from build123d import *

# Parameters (mm, degrees)
SKETCH_1_W          = 80
SKETCH_1_H          = 90
SKETCH_1_R          = 3
SKETCH_1_R_2        = 2
SKETCH_1_W_2        = 20
SKETCH_1_H_2        = 41
EXTRUDE_1_DEPTH     = 5
FILLET_1_R          = 10
SKETCH_2_R          = 1.5
CUT_EXTRUDE_1_DEPTH = 73.284161474


with BuildPart() as part:
    # 草图1 → 凸台-拉伸1 (new body)
    with BuildSketch(Plane(origin=(0, 0, 0), x_dir=(1, 0, 0), z_dir=(0, 1, 0))):
        with Locations((0, 15)):
            Rectangle(SKETCH_1_W, SKETCH_1_H)
        with Locations(Location((27.5, 15, 0), (0, 0, 270))):
            Circle(SKETCH_1_R, mode=Mode.SUBTRACT)
        with Locations(Location((27.5, -15, 0), (0, 0, 270))):
            Circle(SKETCH_1_R, mode=Mode.SUBTRACT)
        with Locations(Location((-27.5, -15, 0), (0, 0, 90))):
            Circle(SKETCH_1_R, mode=Mode.SUBTRACT)
        with Locations(Location((-27.5, 15, 0), (0, 0, 90))):
            Circle(SKETCH_1_R, mode=Mode.SUBTRACT)
        with Locations(Location((4.95, 24.3, 0), (0, 0, 270))):
            Circle(SKETCH_1_R_2, mode=Mode.SUBTRACT)
        with Locations(Location((-4.95, 24.3, 0), (0, 0, 90))):
            Circle(SKETCH_1_R_2, mode=Mode.SUBTRACT)
        with Locations(Location((4.95, -24.3, 0), (0, 0, 90))):
            Circle(SKETCH_1_R_2, mode=Mode.SUBTRACT)
        with Locations(Location((-4.95, -24.3, 0), (0, 0, 270))):
            Circle(SKETCH_1_R_2, mode=Mode.SUBTRACT)
        with Locations(Location((-27.5, 45, 0), (0, 0, 90))):
            Circle(SKETCH_1_R, mode=Mode.SUBTRACT)
        with Locations(Location((27.5, 45, 0), (0, 0, 270))):
            Circle(SKETCH_1_R, mode=Mode.SUBTRACT)
        Rectangle(SKETCH_1_W_2, SKETCH_1_H_2, mode=Mode.SUBTRACT)
    extrude(amount=EXTRUDE_1_DEPTH)

    # 圆角1
    fillet_1_edges = [part.edges().sort_by_distance(p)[0] for p in [
        (40, 2.5, -60),
        (40, 2.5, 30),
        (-40, 2.5, 30),
        (-40, 2.5, -60),
    ]]
    fillet(fillet_1_edges, radius=FILLET_1_R)

    # 草图2 → 切除-拉伸1 (cut, through all)
    with BuildSketch(Plane(origin=(0, 0, 0), x_dir=(1, 0, 0), z_dir=(0, 1, 0))):
        with Locations(Location((0, 54.15, 0), (0, 0, 270))):
            Circle(SKETCH_2_R)
        with Locations(Location((8, 46.15, 0), (0, 0, 270))):
            Circle(SKETCH_2_R)
        with Locations(Location((0, 38.15, 0), (0, 0, 270))):
            Circle(SKETCH_2_R)
        with Locations(Location((-8, 46.15, 0), (0, 0, 270))):
            Circle(SKETCH_2_R)
    extrude(amount=CUT_EXTRUDE_1_DEPTH, mode=Mode.SUBTRACT)


solid = part.part
The model under review builds one solid part; all positions refer to its coordinate system, in mm. A direction names the side the tool comes from. Round coordinates to 2 decimals unless told otherwise and drop trailing zeros. Write each loop counter-clockwise with the first axis right and the second up, starting at its lowest first coordinate (ties: lowest second). Pieces come first, ordered by that corner, then holes. Notation, with made-up numbers: M -37.75,53 L 20.25,53 A23 ccw 20.25,78 Z; hole C 10,-7 d4. An arc over 180 degrees is marked long. Answer as CSV lines item,"result". Start each with the question number.
Q1. Consider section B-B, the plane z = -24.3. Give the boundary of the cut face in (x, y), then the cut area to 3 significant figures.
Q2. Consider section D-D, the plane x = -8. Give the boundary of the cut face in (y, z), then the cut area to 3 significant figures.
Q3. Consider section A-A, the plane x = 27.5. Give the boundary of the cut face in (y, z).
Q4. Consider section C-C, the plane y = 3.05. State how many separate pieces and enclosed holes the cut face has, then the cut area to 3 significant figures.
Q5. The part is to be moulded in two halves that separate along X. For faces 1 (the face through (0, 2, 30)), 2 (the face through (-27.6, 2.5, -12)), 3 (the face through (-40, 2, -15)), say which applies: +X half, -X half, draft (parallel to the pull), parting line (faces both ways), or undercut.
Q6. Wall thickness on line 1 along Z through (x, y) = (-8, 2.1); line 2 along X through (y, z) = (2.2, -15); line 3 along Z through (x, y) = (0, 3.7): over which ranges is each line inside the solid? List them lowest first.
Q7. Tool access review of faces 4 (the face through (0, 2, -20.5)), 5 (the face through (40, 2, -15)): name each direction out of +Z, -Z, +X, -X, +Y, -Y from which nothing blocks a thin tool from reaching the whole face with its end or side.
Result set:
1,outline,"M -40,0 L -6.95,0 L -6.95,5 L -40,5 Z; M -2.95,0 L 2.95,0 L 2.95,5 L -2.95,5 Z; M 6.95,0 L 40,0 L 40,5 L 6.95,5 Z"
1,area,"360 mm²"
2,outline,"M 0,-60 L 5,-60 L 5,-47.65 L 0,-47.65 Z; M 0,-44.65 L 5,-44.65 L 5,-20.5 L 0,-20.5 Z; M 0,20.5 L 5,20.5 L 5,30 L 0,30 Z"
2,area,"230 mm²"
3,outline,"M 0,-60 L 5,-60 L 5,-48 L 0,-48 Z; M 0,-42 L 5,-42 L 5,-18 L 0,-18 Z; M 0,-12 L 5,-12 L 5,12 L 0,12 Z; M 0,18 L 5,18 L 5,30 L 0,30 Z"
4,separate pieces,"1"
4,enclosed holes,"15"
4,area,"6,050 mm²"
5,face 1,"draft"
5,face 2,"undercut"
5,face 3,"-X half"
6,line 1,"z = -60 to -47.65, -44.65 to -20.5, 20.5 to 30"
6,line 2,"x = -40 to -30.5, -24.5 to -10, 10 to 24.5, 30.5 to 40"
6,line 3,"z = -60 to -55.65, -52.65 to -39.65, -36.65 to -20.5, 20.5 to 30"
7,face 4,"+Y, -Y"
7,face 5,"+Z, -Z, +X, +Y, -Y"
